```python
from build123d import *

# Parameters (mm, degrees)
SKETCH1_W           = 31
SKETCH1_H           = 45
SKETCH1_W_2         = 25
SKETCH1_H_2         = 39
BOSS_EXTRUDE1_DEPTH = 60
BOSS_EXTRUDE3_DEPTH = 60
SKETCH3_W           = 8
SKETCH3_H           = 52
CUT_EXTRUDE1_DEPTH  = 9
FILLET1_R           = 10


with BuildPart() as part:
    # Sketch1 → Boss-Extrude1 (new body)
    with BuildSketch(Plane(origin=(0, 0, 0), x_dir=(1, 0, 0), z_dir=(0, 1, 0))):
        Rectangle(SKETCH1_W, SKETCH1_H)
        Rectangle(SKETCH1_W_2, SKETCH1_H_2, mode=Mode.SUBTRACT)
    extrude(amount=BOSS_EXTRUDE1_DEPTH)

    # Sketch5 → Boss-Extrude3 (add)
    with BuildSketch(Plane(origin=(0, 60, 0), x_dir=(1, 0, 0), z_dir=(0, 1, 0))):
        with BuildLine():
            ThreePointArc((-25.5, -136.257439501), (-20.323619098, -135.575956026), (-15.5, -133.577947576))
            Line((-15.5, -133.577947576), (15.5, -133.577947576))
            ThreePointArc((15.5, -133.577947576), (20.323619098, -135.575956026), (25.5, -136.257439501))
            Line((25.5, -136.257439501), (25.5, -132.257439501))
            ThreePointArc((25.5, -132.257439501), (9.5, -116.257439501), (25.5, -100.257439501))
            Line((25.5, -100.257439501), (25.5, -96.257439501))
            ThreePointArc((25.5, -96.257439501), (20.323619098, -96.938922975), (15.5, -98.936931425))
            Line((15.5, -98.936931425), (15.5, -22.5))
            Line((15.5, -22.5), (-15.5, -22.5))
            Line((-15.5, -22.5), (-15.5, -98.936931425))
            ThreePointArc((-15.5, -98.936931425), (-20.323619098, -96.938922975), (-25.5, -96.257439501))
            Line((-25.5, -96.257439501), (-25.5, -100.257439501))
            ThreePointArc((-25.5, -100.257439501), (-9.5, -116.257439501), (-25.5, -132.257439501))
            Line((-25.5, -132.257439501), (-25.5, -136.257439501))
        make_face()
    extrude(amount=-BOSS_EXTRUDE3_DEPTH)

    # Sketch3 → Cut-Extrude1 (cut)
    with BuildSketch(Plane(origin=(0, 0, -22.5), x_dir=(-1, 0, 0), z_dir=(0, 0, -1))):
        with Locations((2.5, 30)):
            Rectangle(SKETCH3_W, SKETCH3_H)
    extrude(amount=-CUT_EXTRUDE1_DEPTH, mode=Mode.SUBTRACT)

    # Fillet1
    fillet1_edges = [part.edges().sort_by_distance(p)[0] for p in [
        (-15.5, 30, 98.936931425),
        (15.5, 30, 98.936931425),
    ]]
    fillet(fillet1_edges, radius=FILLET1_R - 0.0001)  # a hair under: the kernel refuses the full size


solid = part.part
```
Input: part model. Units: mm. Frame: model coordinates. A direction names the side the tool comes from. Round coordinates to 2 decimals unless told otherwise and drop trailing zeros. Write each loop counter-clockwise with the first axis right and the second up, starting at its lowest first coordinate (ties: lowest second). Pieces come first, ordered by that corner, then holes. Notation, with made-up numbers: (81, 17) -> (98, 17) arc R22 cw to (98, 38) -> close; hole circle Ø11 at (44, 49.25). An arc over 180 degrees is marked (long way). Answer as CSV lines item,"result".
1. Reachability of faces 1 (the flat face through (-15.5, 30, 31)), 2 (the cylindrical face through (20.253, 30.42, 135.557)), 3 (the flat face through (12.5, 30, 0)), 4 (the flat face through (-6.5, 30, -21)) from +Z, -Z, +X, -X, +Y, -Y: full face, straight path, thin tool, end or side. Return the list, or none.
Geometry says:
face 1,"-Z, -X, +Y, -Y"
face 2,"+Z, +Y, -Y"
face 3,"+Y, -Y"
face 4,"-Z"
2. Section A-A (x = -4.5). Return the cut outline in (y, z).
Geometry says:
outline,"(0, -22.5) -> (4, -22.5) -> (4, -19.5) -> (0, -19.5) -> close; (0, 19.5) -> (60, 19.5) -> (60, 133.58) -> (0, 133.58) -> close; (56, -22.5) -> (60, -22.5) -> (60, -19.5) -> (56, -19.5) -> close"
3. Mould query, pull axis X, two halves, no side actions, for faces 5 (the flat face through (-25.5, 30, 98)), 6 (the flat face through (25.5, 30, 98)), 7 (the flat face through (-12.5, 30, 0)). Classes: +X half, -X half, draft (parallel to the pull), parting line (faces both ways), or undercut.
Geometry says:
face 5,"-X half"
face 6,"+X half"
face 7,"undercut"
4. Section C-C (x = -18.5). Return the cut outline in (y, z), plus the area to 3 significant figures.
Geometry says:
outline,"(0, 93.4) -> (60, 93.4) -> (60, 101.87) -> (0, 101.87) -> close; (0, 130.64) -> (60, 130.64) -> (60, 134.99) -> (0, 134.99) -> close"
area,"769 mm^2"
5. Ray query, L1, parallel to Z at x = 5.5, y = 7.5; L2, parallel to X at y = 48.5, z = -15.5; L3, parallel to Z at x = -4, y = 48. Return the intervals inside material, ascending. Write a range as [from, to].
Geometry says:
L1,"z = [-22.5, -19.5], [19.5, 133.58]"
L2,"x = [-15.5, -12.5], [12.5, 15.5]"
L3,"z = [19.5, 133.58]"
6. Contact query for flat-ended pins moving along their axis: P1, Ø6, axis at y = 16, z = 60.5, coming from the +X side; P2, Ø15.5, axis at x = -3.5, y = 20.5, coming from the +Z side; P3, Ø2, axis at x = -19, y = 15, coming from the -Z side. Output: stop coordinate, or through.
Geometry says:
P1,"stops at x = 15.5"
P2,"stops at z = 133.58"
P3,"stops at z = 92.87"
7. Section B-B (z = -4). Return the cut outline in (x, y), plus the area to 3 significant figures.
Geometry says:
outline,"(-15.5, 0) -> (-12.5, 0) -> (-12.5, 60) -> (-15.5, 60) -> close; (12.5, 0) -> (15.5, 0) -> (15.5, 60) -> (12.5, 60) -> close"
area,"360 mm^2"
